```python
from build123d import *

# Parameters (mm, degrees)
CYLINDER017_R           = 1.7
CYLINDER017_DEPTH       = 80
CYLINDER017_PITCH_ANGLE = 90
BOX_W                   = 15
BOX_H                   = 20
BOX_DEPTH               = 20


with BuildPart() as taladro_tornillo010:
    # Cylinder017 → Cylinder017 (new body)
    with BuildSketch(Plane.XY):
        Circle(CYLINDER017_R)
    extrude(amount=CYLINDER017_DEPTH)


with BuildPart() as taladro_tornillo010_1:
    # Cylinder017 pitch: moved
    add(taladro_tornillo010.part.rotate(Axis((0, 0, 0), (0, 1, 0)), CYLINDER017_PITCH_ANGLE))


with BuildPart() as taladro_tornillo010_2:
    # Cylinder017 placement: moved
    add(taladro_tornillo010_1.part.moved(Location((-20, 10, 10))))


with BuildPart() as cut:
    # Box → Box (new body)
    with BuildSketch(Plane.XY):
        with Locations((7.5, 10)):
            Rectangle(BOX_W, BOX_H)
    extrude(amount=BOX_DEPTH)

    # Cut: cut Taladro tornillo010
    add(taladro_tornillo010_2.part, mode=Mode.SUBTRACT)


solid = cut.part
```
Source: CAD feature listing. Evaluate the final solid. Frame: model axes, mm. Round coordinates to 2 decimals unless told otherwise and drop trailing zeros. Order: outer loops, then holes, each group sorted by start corner. A loop starts at its lowest first (then second) coordinate and runs counter-clockwise, first axis right, second up. Notation, with made-up numbers: (-32, 36.5) -> (23, 36.5) arc R14 cw to (23, 42.5) -> close; hole circle Ø11 at (-2, 82). An arc over 180 degrees is marked (long way). One line per item, written item: value. Start each with the question number.
Q1. Section query C-C (x = 7.5). Return the cut outline in (y, z).
Q2. Material intervals for probe 1 along Y at (x, z) = (11.5, 10); probe 2 along Y at (x, z) = (4.25, 9.5), sorted ascending.
Q3. Pin query (flat end, axial travel): pin 1 (3 mm diameter, centred on y = 10, z = 10, fed in from -X). Return the tip coordinate at first contact, or that it passes through.
Q4. Section query A-A (z = 10). Return the cut outline in (x, y).
Q5. Draft query along Z for faces 1 (the flat face through (0, 12, 10)), 2 (the cylindrical face through (7.4, 9.35, 8.43)), 3 (the flat face through (7, 10, 20)). Return one class per face: pulls with the +Z half, pulls with the -Z half, needs draft (parallel to the pull), parting line crosses it, or undercut.
Findings below:
1. outline: (0, 0) -> (20, 0) -> (20, 20) -> (0, 20) -> close; hole circle Ø3.4 at (10, 10)
2. probe 1: 0 to 8.3, 11.7 to 20
2. probe 2: 0 to 8.38, 11.62 to 20
3. pin 1: through
4. outline: (0, 0) -> (15, 0) -> (15, 8.3) -> (0, 8.3) -> close; (0, 11.7) -> (15, 11.7) -> (15, 20) -> (0, 20) -> close
5. face 1: needs draft
5. face 2: undercut
5. face 3: pulls with the +Z half
